from build123d import *

# Parameters (mm, degrees)
SKETCH2_W           = 152.4
SKETCH2_H           = 76.2
BOSS_EXTRUDE2_DEPTH = 6.35
SKETCH3_W           = 139.7
SKETCH3_H           = 63.5
CUT_EXTRUDE1_DEPTH  = 6.35
SKETCH4_W           = 6.35
SKETCH4_H           = 6.35
BOSS_EXTRUDE3_DEPTH = 12.7


with BuildPart() as part:
    # Sketch2 → Boss-Extrude2 (new body)
    with BuildSketch(Plane(origin=(0, 0, 0), x_dir=(1, 0, 0), z_dir=(0, 1, 0))):
        Rectangle(SKETCH2_W, SKETCH2_H)
    extrude(amount=-BOSS_EXTRUDE2_DEPTH)

    # Sketch3 → Cut-Extrude1 (cut)
    with BuildSketch(Plane(origin=(0, -6.35, 0), x_dir=(-1, 0, 0), z_dir=(0, -1, 0))):
        Rectangle(SKETCH3_W, SKETCH3_H)
    extrude(amount=-CUT_EXTRUDE1_DEPTH, mode=Mode.SUBTRACT)

    # Sketch4 → Boss-Extrude3 (add)
    with BuildSketch(Plane(origin=(0, 0, 0), x_dir=(1, 0, 0), z_dir=(0, 1, 0))):
        with Locations((-73.025, 34.925)):
            Rectangle(SKETCH4_W, SKETCH4_H)
        with Locations((-73.025, -34.925)):
            Rectangle(SKETCH4_W, SKETCH4_H)
        with Locations((73.025, -34.925)):
            Rectangle(SKETCH4_W, SKETCH4_H)
        with Locations((73.025, 34.925)):
            Rectangle(SKETCH4_W, SKETCH4_H)
    extrude(amount=BOSS_EXTRUDE3_DEPTH)


solid = part.part
Check sheet for the modelled part. Datum: model origin and axes. Units: mm. A direction names the side the tool comes from. Round coordinates to 2 decimals unless told otherwise and drop trailing zeros. Loops run counter-clockwise (first coordinate to the right, second up) from the corner with the lowest first, then second, coordinate; pieces in that order, holes last.
1. Sectioned sample at A-A on x = 50. Record the boundary of the cut face in (y, z).
2. Gauge pin test, flat end, axial feed: pin 1 Ø5 at (x, z) = (74.5, -7) entering from +Y. Record the tip position at first contact, or that the pin passes through.
3. Mould release check, pull along X, two halves, no side actions. Record for faces 5 (the flat face through (-73, 12.7, 35)), 6 (the flat face through (69.85, 6, -35)), 7 (the flat face through (76.2, -1, 1)): released by +X, released by -X, zero draft, split by the parting line, or undercut.
4. Sectioned sample at B-B on z = 11. Record the boundary of the cut face in (x, y).
5. Sectioned sample at C-C on y = 5.75. Record the boundary of the cut face in (x, z), and give its area (3 significant figures).
6. Set-up check for faces 1 (the flat face through (-73, 0, 0)), 2 (the flat face through (-6, -6.35, 34)), 3 (the flat face through (69.85, 6, 35)), 4 (the flat face through (1, -3, -31.75)): record each of +Z, -Z, +X, -X, +Y, -Y from which the full face is reachable in a straight line by a thin tool's end or side.
7. Scan lines: probe 1 along X at (y, z) = (-3.5, -8.5); probe 2 along Z at (x, y) = (20, -4.25); probe 3 along Y at (x, z) = (70, -2). Record each from-to range of solid material in increasing order.
8. Sectioned sample at D-D on y = -3.75. Record the boundary of the cut face in (x, z).
Recorded:
1. outline: (-6.35, -38.1) - (0, -38.1) - (0, -31.75) - (-6.35, -31.75) - close; (-6.35, 31.75) - (0, 31.75) - (0, 38.1) - (-6.35, 38.1) - close
2. pin 1: stops at y = 0
3. face 5: zero draft
3. face 6: undercut
3. face 7: released by +X
4. outline: (-76.2, -6.35) - (-69.85, -6.35) - (-69.85, 0) - (-76.2, 0) - close; (69.85, -6.35) - (76.2, -6.35) - (76.2, 0) - (69.85, 0) - close
5. outline: (-76.2, -38.1) - (-69.85, -38.1) - (-69.85, -31.75) - (-76.2, -31.75) - close; (-76.2, 31.75) - (-69.85, 31.75) - (-69.85, 38.1) - (-76.2, 38.1) - close; (69.85, -38.1) - (76.2, -38.1) - (76.2, -31.75) - (69.85, -31.75) - close; (69.85, 31.75) - (76.2, 31.75) - (76.2, 38.1) - (69.85, 38.1) - close
5. area: 161 mm2
6. face 1: +X, -X, +Y
6. face 2: +Z, -Z, +X, -X, -Y
6. face 3: +Z, -Z, +Y
6. face 4: +Y, -Y
7. probe 1: x = -76.2 to -69.85, 69.85 to 76.2
7. probe 2: z = -38.1 to -31.75, 31.75 to 38.1
7. probe 3: y = -6.35 to 0
8. outline: (-76.2, -38.1) - (76.2, -38.1) - (76.2, 38.1) - (-76.2, 38.1) - close; hole (-69.85, -31.75) - (69.85, -31.75) - (69.85, 31.75) - (-69.85, 31.75) - close
